Source: CAD feature listing. Evaluate the final solid. Frame: model axes, mm. A direction names the side the tool comes from. Round coordinates to 2 decimals unless told otherwise and drop trailing zeros. Write each loop counter-clockwise with the first axis right and the second up, starting at its lowest first coordinate (ties: lowest second). Pieces come first, ordered by that corner, then holes.
from build123d import *

# Parameters (mm, degrees)
FILLET1_R    = 0.2
SKETCH3_W    = 1.03
SKETCH3_H    = 4.3
SKETCH4_W    = 1.03
SKETCH4_H    = 1.966638464
RECPAT_COUNT = 2
RECPAT_ANGLE = 90


with BuildPart() as part:
    # BodySke → Base-Revolve (revolve)
    with BuildSketch(Plane.XY):
        with BuildLine():
            Line((3.1, 2), (3.1, 4))
            Line((3.1, 4), (1.555305874, 4))
            ThreePointArc((1.555305874, 4), (1.392873227, 3.961271902), (1.265388955, 3.853420195))
            ThreePointArc((1.265388955, 3.853420195), (0.324444487, 2.027933456), (0, 0))
            Line((0, 0), (13.1, 0))
            Line((13.1, 0), (13.1, 2))
            Line((13.1, 2), (3.1, 2))
        make_face()
    revolve(axis=Axis((-25.4, 0, 0), (1, 0, 0)))

    # Fillet1
    fillet1_edges = [part.edges().sort_by_distance(p)[0] for p in [
        (3.1, -2, 0),
    ]]
    fillet(fillet1_edges, radius=FILLET1_R)

    # Sketch3 → Recess section 0
    with BuildSketch(Plane(origin=(0, 0, 0), x_dir=(0, 0, -1), z_dir=(1, 0, 0))):
        Rectangle(SKETCH3_W, SKETCH3_H)
    # Sketch4 → Recess section 1
    with BuildSketch(Plane(origin=(2.34, 0, 0), x_dir=(0, 0, -1), z_dir=(1, 0, 0))):
        Rectangle(SKETCH4_W, SKETCH4_H)
    recess = loft(mode=Mode.SUBTRACT)

    # RecPat: Recess ×2 about axis
    recpat_axis = Axis((0, 0, 0), (1, 0, 0))
    for i in range(1, RECPAT_COUNT):
        add(recess.rotate(recpat_axis, i * RECPAT_ANGLE / (RECPAT_COUNT - 1)), mode=Mode.SUBTRACT)

    # RecCorSke → RecessCore (revolve, cut)
    with BuildSketch(Plane.XY):
        Polygon((0, 0), (0, 1.01462874), (2.34, 0.851), (2.616506661, 0), align=None)
    revolve(axis=Axis((-3.175, 0, 0), (1, 0, 0)), mode=Mode.SUBTRACT)


solid = part.part
1) Section query A-A on x = 3.5. Return the cut outline in (y, z), then the cut area to 3 significant figures.
Taken from the geometry:
outline: circle Ø4 at (0, 0)
area: 12.6 mm2
2) Pull-direction query (Y, two-part tool) for faces 1 (the face through (3.1, -2, -2)), 2 (the face through (1.3, 1.5, 0)), 3 (the face through (2.317, -0.867, -3.905)); classes: released by +Y, released by -Y, zero draft, split by the parting line, or undercut.
Taken from the geometry:
face 1: zero draft
face 2: undercut
face 3: split by the parting line
3) Contact query for flat-ended pins moving along their axis: P1, Ø1.5, axis at x = 11.5, z = -1, coming from the +Y side; P2, Ø4, axis at y = 3, z = -1.5, coming from the -X side; P3, Ø2, axis at x = 5, y = 2, coming from the +Z side. Output: stop coordinate, or through.
Taken from the geometry:
P1: stops at y = 1.98
P2: stops at x = 0.14
P3: stops at z = 1.73
4) Material intervals for line 1 (Y direction, x = 1, z = 0.25); line 2 (X direction, y = -3.25, z = -0.5); line 3 (Y direction, x = 10.5, z = 1.75), sorted ascending.
Taken from the geometry:
line 1: y = -3.46 to -1.65, 1.65 to 3.46
line 2: x = 0.89 to 3.1
line 3: y = -0.97 to 0.97
5) Reachability of faces 4 (the face through (1.3, 0, 1.5)), 5 (the face through (8, 0, -2)), 6 (the face through (13.1, 0, 0)) from +Z, -Z, +X, -X, +Y, -Y: full face, straight path, thin tool, end or side. Return the list, or none.
Taken from the geometry:
face 4: -X
face 5: +X
face 6: +Z, -Z, +X, +Y, -Y
